The listing builds one solid part. Answer for the finished solid, in the listing's coordinates (mm). A direction names the side the tool comes from. Round coordinates to 2 decimals unless told otherwise and drop trailing zeros. Write each loop counter-clockwise with the first axis right and the second up, starting at its lowest first coordinate (ties: lowest second). Pieces come first, ordered by that corner, then holes.
from build123d import *

# Parameters (mm, degrees)
SKETCH1_W               = 55
SKETCH1_H               = 70
BOSS_EXTRUDE1_DEPTH     = 4
SKETCH4_W               = 26
SKETCH4_H               = 25
BOSS_EXTRUDE2_DEPTH     = 2
SKETCH3_R               = 4.1
CUT_EXTRUDE1_DEPTH      = 22
SKETCH5_W               = 40
SKETCH5_H               = 45
BOSS_EXTRUDE3_DEPTH     = 4
SKETCH7_R               = 11.3
SKETCH7_R_2             = 1.5
CUT_EXTRUDE2_DEPTH      = 77.270898775
FILLET1_R               = 4
SKETCH8_W               = 4
SKETCH8_H               = 25
BOSS_EXTRUDE4_DEPTH     = 4
FILLET2_R               = 4
SKETCH10_W              = 69
SKETCH10_H              = 3
BOSS_EXTRUDE5_DEPTH     = 6
CUT_EXTRUDE4_DEPTH      = 77.270898775
CUT_EXTRUDE4_DEPTH_BACK = 77.270898775
SKETCH12_R              = 1.65
CUT_EXTRUDE5_DEPTH      = 77.689308251
CUT_EXTRUDE5_DEPTH_BACK = 77.689308251
SKETCH13_R              = 1.65
FILLET3_R               = 4


with BuildPart() as part:
    # Sketch1 → Boss-Extrude1 (new body)
    with BuildSketch(Plane.XY):
        Rectangle(SKETCH1_W, SKETCH1_H)
    extrude(amount=BOSS_EXTRUDE1_DEPTH)

    # Sketch4 → Boss-Extrude2 (add)
    with BuildSketch(Plane.XY.offset(4)):
        with Locations((-14.5, 20)):
            Rectangle(SKETCH4_W, SKETCH4_H)
        with Locations((-14.5, -20)):
            Rectangle(SKETCH4_W, SKETCH4_H)
    extrude(amount=BOSS_EXTRUDE2_DEPTH)

    # Sketch3 → Cut-Extrude1 (cut)
    with BuildSketch(Plane.ZY.offset(27.5)):
        with Locations((6.1, 20)):
            Circle(SKETCH3_R)
        with Locations((6.1, -20)):
            Circle(SKETCH3_R)
    extrude(amount=-CUT_EXTRUDE1_DEPTH, mode=Mode.SUBTRACT)

    # Sketch5 → Boss-Extrude3 (add)
    with BuildSketch(Plane.XY.offset(4)):
        with Locations((47.5, 0)):
            Rectangle(SKETCH5_W, SKETCH5_H)
    extrude(amount=-BOSS_EXTRUDE3_DEPTH)

    # Sketch7 → Cut-Extrude2 (cut, through all)
    with BuildSketch(Plane(origin=(0, 0, 0), x_dir=(-1, 0, 0), z_dir=(0, 0, -1))):
        with Locations((-44.5, 0)):
            Circle(SKETCH7_R)
        with Locations((-60, 15.5)):
            Circle(SKETCH7_R_2)
        with Locations((-29, 15.5)):
            Circle(SKETCH7_R_2)
        with Locations((-29, -15.5)):
            Circle(SKETCH7_R_2)
        with Locations((-60, -15.5)):
            Circle(SKETCH7_R_2)
    extrude(amount=-CUT_EXTRUDE2_DEPTH, mode=Mode.SUBTRACT)

    # Fillet1
    fillet1_edges = [part.edges().sort_by_distance(p)[0] for p in [
        (27.5, -35, 2),
        (27.5, 35, 2),
    ]]
    fillet(fillet1_edges, radius=FILLET1_R)

    # Sketch8 → Boss-Extrude4 (add)
    with BuildSketch(Plane.XY.offset(6)):
        with Locations((-3.5, 20)):
            Rectangle(SKETCH8_W, SKETCH8_H)
        with Locations((-3.5, -20)):
            Rectangle(SKETCH8_W, SKETCH8_H)
    extrude(amount=BOSS_EXTRUDE4_DEPTH)

    # Fillet2
    fillet2_edges = [part.edges().sort_by_distance(p)[0] for p in [
        (-3.5, -32.5, 10),
        (-3.5, -7.5, 10),
        (-3.5, 32.5, 10),
        (-3.5, 7.5, 10),
    ]]
    fillet(fillet2_edges, radius=FILLET2_R)

    # Sketch10 → Boss-Extrude5 (add)
    with BuildSketch(Plane.XY.offset(4)):
        with Locations((33, 21)):
            Rectangle(SKETCH10_W, SKETCH10_H)
        with Locations((33, -21)):
            Rectangle(SKETCH10_W, SKETCH10_H)
    extrude(amount=BOSS_EXTRUDE5_DEPTH)

    # Sketch12 → Cut-Extrude4 (cut, two sides: drawn at the far end of the back side and taken through both)
    with BuildSketch(Plane.XY.offset(4).offset(-CUT_EXTRUDE4_DEPTH_BACK)):
        with Locations((3.466076719, 28.5)):
            Circle(SKETCH12_R)
        with Locations((24, 28.5)):
            Circle(SKETCH12_R)
        with Locations((24.385, -28.5)):
            Circle(SKETCH12_R)
        with Locations((3.081076719, -28.5)):
            Circle(SKETCH12_R)
    extrude(amount=CUT_EXTRUDE4_DEPTH + CUT_EXTRUDE4_DEPTH_BACK, mode=Mode.SUBTRACT)

    # Sketch13 → Cut-Extrude5 (cut, two sides: drawn at the far end of the back side and taken through both)
    with BuildSketch(Plane(origin=(0, 0, 0), x_dir=(-1, 0, 0), z_dir=(0, 0, -1)).offset(-CUT_EXTRUDE5_DEPTH_BACK)):
        with Locations(Location((21, -11.761910465, 0), (0, 0, 180))):
            Circle(SKETCH13_R)
        with Locations(Location((21, -28.238089535, 0), (0, 0, 180))):
            Circle(SKETCH13_R)
        with Locations((21, 28.238089535)):
            Circle(SKETCH13_R)
        with Locations((21, 11.761910465)):
            Circle(SKETCH13_R)
    extrude(amount=CUT_EXTRUDE5_DEPTH + CUT_EXTRUDE5_DEPTH_BACK, mode=Mode.SUBTRACT)

    # Fillet3
    fillet3_edges = [part.edges().sort_by_distance(p)[0] for p in [
        (67.5, 22.5, 5),
        (67.5, -22.5, 5),
    ]]
    fillet(fillet3_edges, radius=FILLET3_R)


solid = part.part
1. Section B-B on x = 60 is taken. Determine the outline of the cut face in (y, z).
Geometry says:
outline: (-22.5, 0) - (-17, 0) - (-17, 4) - (-19.5, 4) - (-19.5, 10) - (-22.5, 10) - close; (-14, 0) - (14, 0) - (14, 4) - (-14, 4) - close; (17, 0) - (22.5, 0) - (22.5, 10) - (19.5, 10) - (19.5, 4) - (17, 4) - close
2. Given pin 1 (1.8 mm diameter, centred on y = -13, z = 6, fed in from +X); pin 2 (9 mm diameter, centred on x = -11.5, y = 12, fed in from +Z); pin 3 (3 mm diameter, centred on x = 34.5, z = 9, fed in from -Y); pin 4 (1.8 mm diameter, centred on x = 60, y = 15.5, fed in from +Z), each flat-ended and moving along its own axis, determine where each tip first touches the part or whether it passes through.
Geometry says:
pin 1: stops at x = -1.5
pin 2: stops at z = 6
pin 3: stops at y = -22.5
pin 4: passes through
3. For a pull along Y with two mould halves and no side action, classify faces 4 (the face through (33.72, 3.39, 1.97)), 5 (the face through (-17, 20, 2)), 6 (the face through (-17, -28, 6)), 7 (the face through (26.297, 33.859, 2.028)) as released by +Y, released by -Y, zero draft, split by the parting line, or undercut.
Geometry says:
face 4: undercut
face 5: undercut
face 6: zero draft
face 7: released by +Y
4. Section C-C on z = 7.25 is taken. Determine the outline of the cut face in (x, y), plus the area to 3 significant figures.
Geometry says:
outline: (-5.5, -32.3) - (-1.5, -32.3) - (-1.5, -22.5) - (63.5, -22.5) arc R4 ccw to (67.37, -19.5) - (-1.5, -19.5) - (-1.5, -7.7) - (-5.5, -7.7) - close; (-5.5, 7.7) - (-1.5, 7.7) - (-1.5, 19.5) - (67.37, 19.5) arc R4 ccw to (63.5, 22.5) - (-1.5, 22.5) - (-1.5, 32.3) - (-5.5, 32.3) - close
area: 604 mm2
5. Section A-A on x = -21 is taken. Give the number of separate pieces and of enclosed holes in the cut face, plus the area to 3 significant figures.
Geometry says:
separate pieces: 5
enclosed holes: 0
area: 250 mm2
6. A tool of negligible diameter and unlimited length cuts with its end or side. For faces 1 (the face through (-15, -7.5, 5)), 2 (the face through (-5.5, 20, 7)), 3 (the face through (27.5, 27, 2)), from which of +Z, -Z, +X, -X, +Y, -Y can it reach the whole face along a straight path? Write none if from no direction.
Geometry says:
face 1: +Z, +X, -X
face 2: +Z, -X
face 3: +Z, -Z, +X, +Y
7. Straight lines are drawn through the part: line 1 along Y through (x, z) = (29, 1.8); line 2 along X through (y, z) = (28.5, 2.45); line 3 along Y through (x, z) = (-21, 1.5). For each, find the intervals that lie inside material, in ascending order.
Geometry says:
line 1: y = -22.5 to -17, -14 to 14, 17 to 22.5
line 2: x = -27.5 to -22.63, -19.37 to 1.82, 5.12 to 22.35, 25.65 to 27.5
line 3: y = -35 to -29.89, -26.59 to -13.41, -10.11 to 10.11, 13.41 to 26.59, 29.89 to 35
8. Section D-D on x = 44.5 is taken. Determine the outline of the cut face in (y, z).
Geometry says:
outline: (-22.5, 0) - (-11.3, 0) - (-11.3, 4) - (-19.5, 4) - (-19.5, 10) - (-22.5, 10) - close; (11.3, 0) - (22.5, 0) - (22.5, 10) - (19.5, 10) - (19.5, 4) - (11.3, 4) - close
